Here's how the part is built. I have some questions about the finished solid (model axes, mm). Coordinates: 2 decimals unless noted, no trailing zeros. Loops run counter-clockwise (first coordinate to the right, second up) from the corner with the lowest first, then second, coordinate; pieces in that order, holes last. Notation, with made-up numbers: M -36.75,-31 L -16.75,-31 A23 cw -16.75,-8 Z; hole C 38,45 d5. An arc over 180 degrees is marked long. Use CSV: the item, a comma, the result in double quotes. Start each with the question number.
Q1. If we section it at C-C (y = 2.7): State how many separate pieces and enclosed holes the cut face has, and give its area (3 significant figures).
Q2. If we section it at D-D (z = -22): Please give me the cut outline in (x, y).
Q3. If we section it at B-B (x = 29.5): Please give me the cut outline in (y, z).
Q4. For pin 1 Ø2 at (x, y) = (-16.5, 2.5) entering from +Z; pin 2 Ø2 at (x, y) = (23, 1.5) entering from +Z; pin 3 Ø1 at (x, y) = (-25, 2) entering from -Z, each with a flat end and sliding along its axis, tell me the tip position at first contact or that it passes through.
Q5. Please list where these lines run through material, in increasing order: probe 1 along X at (y, z) = (0.2, -16); probe 2 along X at (y, z) = (2.1, 28.5); probe 3 along Z at (x, y) = (-5, 2.25). Write a range as [from, to].
Q6. If we mould it in two halves opening along X, with no side actions, what happens to faces 1 (the cylindrical face through (-32.28, 1.97, -13.57)), 2 (the flat face through (23.48, 2.03, -22.7)), 3 (the cylindrical face through (-27.914, 2.028, 3.792)), 4 (the flat face through (0, 0, 0))? For each: +X half, -X half, draft (parallel to the pull), parting line (faces both ways), or undercut.
Q7. If we section it at A-A (z = 28.5): Please give me the cut outline in (x, y).
from build123d import *

# Parameters (mm, degrees)
SKETCH_1_W          = 65
SKETCH_1_H          = 63
EXTRUDE_1_DEPTH     = 4
SKETCH_2_R          = 1.6
CUT_EXTRUDE_1_DEPTH = 4
SKETCH_3_R          = 1.6
CUT_EXTRUDE_2_DEPTH = 4
FILLET_1_R          = 3
CUT_EXTRUDE_3_DEPTH = 10
FILLET_2_R          = 3


with BuildPart() as part:
    # 草图1 → 凸台-拉伸1 (new body)
    with BuildSketch(Plane(origin=(0, 0, 0), x_dir=(1, 0, 0), z_dir=(0, 1, 0))):
        Rectangle(SKETCH_1_W, SKETCH_1_H)
    extrude(amount=EXTRUDE_1_DEPTH)

    # 草图2 → 切除-拉伸1 (cut)
    with BuildSketch(Plane(origin=(0, 4, 0), x_dir=(1, 0, 0), z_dir=(0, 1, 0))):
        with Locations(Location((-15, -15, 0), (0, 0, 270))):
            Circle(SKETCH_2_R)
        with Locations(Location((-15, 15, 0), (0, 0, 90))):
            Circle(SKETCH_2_R)
        with Locations(Location((15, 15, 0), (0, 0, 270))):
            Circle(SKETCH_2_R)
        with Locations(Location((15, -15, 0), (0, 0, 90))):
            Circle(SKETCH_2_R)
    extrude(amount=-CUT_EXTRUDE_1_DEPTH, mode=Mode.SUBTRACT)

    # 草图3 → 切除-拉伸2 (cut)
    with BuildSketch(Plane(origin=(0, 4, 0), x_dir=(1, 0, 0), z_dir=(0, 1, 0))):
        with Locations(Location((-4, -28.5, 0), (0, 0, 270))):
            Circle(SKETCH_3_R)
        with Locations(Location((4, -28.5, 0), (0, 0, 90))):
            Circle(SKETCH_3_R)
        with Locations(Location((4, 28.5, 0), (0, 0, 270))):
            Circle(SKETCH_3_R)
        with Locations(Location((-4, 28.5, 0), (0, 0, 90))):
            Circle(SKETCH_3_R)
        with Locations(Location((-29.5, -4, 0), (0, 0, 270))):
            Circle(SKETCH_3_R)
        with Locations(Location((-29.5, 4, 0), (0, 0, 90))):
            Circle(SKETCH_3_R)
        with Locations(Location((29.5, 4, 0), (0, 0, 270))):
            Circle(SKETCH_3_R)
        with Locations(Location((29.5, -4, 0), (0, 0, 90))):
            Circle(SKETCH_3_R)
    extrude(amount=-CUT_EXTRUDE_2_DEPTH, mode=Mode.SUBTRACT)

    # 圆角1
    fillet_1_edges = [part.edges().sort_by_distance(p)[0] for p in [
        (32.5, 2, 31.5),
        (-32.5, 2, 31.5),
        (-32.5, 2, -31.5),
        (32.5, 2, -31.5),
    ]]
    fillet(fillet_1_edges, radius=FILLET_1_R)

    # 草图5 → 切除-拉伸3 (cut)
    with BuildSketch(Plane(origin=(0, 4, 0), x_dir=(1, 0, 0), z_dir=(0, 1, 0))):
        Polygon((-47.682171846, -46.682171846), (-9.681789184, -36.5), (-37.5, -8.681789184), align=None)
        Polygon((37.5, -8.681789184), (47.682171846, -46.682171846), (9.681789184, -36.5), align=None)
        Polygon((-37.5, 8.681789184), (-47.682171846, 46.682171846), (-9.681789184, 36.5), align=None)
        Polygon((37.5, 8.681789184), (47.682171846, 46.682171846), (9.681789184, 36.5), align=None)
    extrude(amount=-CUT_EXTRUDE_3_DEPTH, mode=Mode.SUBTRACT)

    # 圆角2
    fillet_2_edges = [part.edges().sort_by_distance(p)[0] for p in [
        (32.5, 2, 13.681789184),
        (14.681789184, 2, 31.5),
        (-14.681789184, 2, -31.5),
        (-32.5, 2, -13.681789184),
        (32.5, 2, -13.681789184),
        (14.681789184, 2, -31.5),
        (-32.5, 2, 13.681789184),
        (-14.681789184, 2, 31.5),
    ]]
    fillet(fillet_2_edges, radius=FILLET_2_R)


solid = part.part
Results below:
1,separate pieces,"1"
1,enclosed holes,"12"
1,area,"3,360 mm^2"
2,outline,"M -24.18,0 L 24.18,0 L 24.18,4 L -24.18,4 Z"
3,outline,"M 0,-16.68 L 4,-16.68 L 4,-5.6 L 0,-5.6 Z; M 0,-2.4 L 4,-2.4 L 4,2.4 L 0,2.4 Z; M 0,5.6 L 4,5.6 L 4,16.68 L 0,16.68 Z"
4,pin 1,"z = 30.68"
4,pin 2,"z = 24.18"
4,pin 3,"z = -21.68"
5,probe 1,"[-30.18, -16.25], [-13.75, 13.75], [16.25, 30.18]"
5,probe 2,"[-17.68, -5.6], [-2.4, 2.4], [5.6, 17.68]"
5,probe 3,"[-31.5, -29.75], [-27.25, 27.25], [29.75, 31.5]"
6,face 1,"-X half"
6,face 2,"+X half"
6,face 3,"undercut"
6,face 4,"draft"
7,outline,"M -17.68,0 L -5.6,0 L -5.6,4 L -17.68,4 Z; M -2.4,0 L 2.4,0 L 2.4,4 L -2.4,4 Z; M 5.6,0 L 17.68,0 L 17.68,4 L 5.6,4 Z"
